```python
from build123d import *


with BuildPart() as part:
    # 扫描1: sweep along a path in 草图1
    with BuildLine(Plane.XY) as sweep_1_path:
        Line((-90, 16), (130, 16))
        ThreePointArc((130, 16), (146, 0), (130, -16))
        Line((130, -16), (-90, -16))
        ThreePointArc((-90, -16), (-106, 0), (-90, 16))
    # 草图2 → 扫描1 (sweep)
    with BuildSketch(Plane(origin=(0, 0, 0), x_dir=(1, 0, 0), z_dir=(0, 1, 0))):
        Polygon((-106, 0), (-106, 4.5), (-103.4, 2.25), (-103.4, -2.25), (-106, -4.5), align=None)
    sweep(path=sweep_1_path.line)


solid = part.part
```
Part model, mm, in its own coordinate system. A direction names the side the tool comes from. Round coordinates to 2 decimals unless told otherwise and drop trailing zeros. Loops run counter-clockwise (first coordinate to the right, second up) from the corner with the lowest first, then second, coordinate; pieces in that order, holes last. Notation, with made-up numbers: (86, 24) -> (131, 24) arc R14 ccw to (131, 40) -> close; hole circle Ø6 at (-7, -18.5). An arc over 180 degrees is marked (long way). Use CSV: the item, a comma, the result in double quotes. Start each with the question number.
1) Wall check: L1, parallel to Y at x = 75.5, z = 0; L2, parallel to X at y = -1, z = -0.5; L3, parallel to X at y = -4.5, z = -3.5. Give the ranges that are in metal, low to high. Write a range as [from, to].
2) Pull direction Y, two halves, no side cores. Call faces 6 (the flat face through (22, 16, 0)), 7 (the flat face through (18, -16, 0)), 8 (the cylindrical face through (143.397, 0.295, -0.031)), 9 (the conical face through (-103.523, -0.297, 2.359)): +Y half, -Y half, draft (parallel to the pull), parting line (faces both ways), or undercut.
3) Drop flat-ended pins along their axis: P1, Ø3, axis at y = -7.5, z = 1, coming from the +X side; P2, Ø3, axis at y = 4.5, z = -2.5, coming from the -X side; P3, Ø3, axis at x = 17.5, y = -11.5, coming from the +Z side. Give the stop position or say it passes through.
4) Cut at B-B, the plane x = 120.5. Write the cut outline in (y, z).
5) Cut at A-A, the plane y = 0. Write the cut outline in (x, z), plus the area to 3 significant figures.
6) Which spindle directions (+Z, -Z, +X, -X, +Y, -Y) get a long thin tool onto all of the face, cutting with end or side? Do faces 1 (the cylindrical face through (-106, 0, 0)), 2 (the cylindrical face through (146, 0, 0)), 3 (the flat face through (22, 13.4, 0)), 4 (the conical face through (143.523, 0.297, 2.359)), 5 (the conical face through (143.56, 0.3, -2.39)). Say none if no direction does.
Determined:
1,L1,"y = [-16, -13.4], [13.4, 16]"
1,L2,"x = [-105.97, -103.36], [143.36, 145.97]"
1,L3,"x = [-105.35, -104.15], [144.15, 145.35]"
2,face 6,"+Y half"
2,face 7,"-Y half"
2,face 8,"undercut"
2,face 9,"undercut"
3,P1,"stops at x = 144.83"
3,P2,"stops at x = -105.72"
3,P3,"passes through"
4,outline,"(-16, -4.5) -> (-13.4, -2.25) -> (-13.4, 2.25) -> (-16, 4.5) -> close; (13.4, -2.25) -> (16, -4.5) -> (16, 4.5) -> (13.4, 2.25) -> close"
5,outline,"(-106, -4.5) -> (-103.4, -2.25) -> (-103.4, 2.25) -> (-106, 4.5) -> close; (143.4, -2.25) -> (146, -4.5) -> (146, 4.5) -> (143.4, 2.25) -> close"
5,area,"35.1 mm2"
6,face 1,"+Z, -Z, -X"
6,face 2,"+Z, -Z, +X"
6,face 3,"+Z, -Z"
6,face 4,"+Z"
6,face 5,"-Z"
